Build history of the part. All positions in model axes, mm. Round coordinates to 2 decimals unless told otherwise and drop trailing zeros. Write each loop counter-clockwise with the first axis right and the second up, starting at its lowest first coordinate (ties: lowest second). Pieces come first, ordered by that corner, then holes.
1) Flat gauge pins, fed straight in: pin 1 (1.5 mm diameter, centred on x = 62.5, y = 0.5, fed in from +Z); pin 2 (2.5 mm diameter, centred on x = -95, z = 0, fed in from -Y). Where does each tip first touch, or does it go through?
2) Saw through at B-B (x = -119). Write the cut outline in (y, z), plus the area to 3 significant figures.
3) Saw through at C-C (z = 106). Write the cut outline in (x, y).
4) Wall check: probe 1 along X at (y, z) = (1.25, 0.5); probe 2 along Z at (x, y) = (-95, 0.75); probe 3 along X at (y, z) = (1.6, -45). Give the ranges that are in metal, low to high.
5) Saw through at A-A (y = 2.15). State how many separate pieces and enclosed holes the cut face has, plus the area to 3 significant figures.
from build123d import *

# Parameters (mm, degrees)
SKETCH1_R           = 150
SKETCH1_R_2         = 2.45
SKETCH1_R_3         = 1.45
BOSS_EXTRUDE1_DEPTH = 3


with BuildPart() as part:
    # Sketch1 → Boss-Extrude1 (new body)
    with BuildSketch(Plane(origin=(0, 0, 0), x_dir=(1, 0, 0), z_dir=(0, 1, 0))):
        with Locations(Location((0, 0, 0), (0, 0, 270))):
            Circle(SKETCH1_R)
        with Locations(Location((0, 10, 0), (0, 0, 270))):
            Circle(SKETCH1_R_2, mode=Mode.SUBTRACT)
        with Locations(Location((0, -10, 0), (0, 0, 270))):
            Circle(SKETCH1_R_2, mode=Mode.SUBTRACT)
        with Locations(Location((45, 0, 0), (0, 0, 270))):
            Circle(SKETCH1_R_3, mode=Mode.SUBTRACT)
        with Locations(Location((95, 0, 0), (0, 0, 270))):
            Circle(SKETCH1_R_3, mode=Mode.SUBTRACT)
        with Locations(Location((0, -45, 0), (0, 0, 270))):
            Circle(SKETCH1_R_3, mode=Mode.SUBTRACT)
        with Locations(Location((0, -95, 0), (0, 0, 270))):
            Circle(SKETCH1_R_3, mode=Mode.SUBTRACT)
        with Locations(Location((-95, 0, 0), (0, 0, 270))):
            Circle(SKETCH1_R_3, mode=Mode.SUBTRACT)
        with Locations(Location((-45, 0, 0), (0, 0, 270))):
            Circle(SKETCH1_R_3, mode=Mode.SUBTRACT)
        with Locations(Location((0, 95, 0), (0, 0, 270))):
            Circle(SKETCH1_R_3, mode=Mode.SUBTRACT)
        with Locations(Location((0, 45, 0), (0, 0, 270))):
            Circle(SKETCH1_R_3, mode=Mode.SUBTRACT)
    extrude(amount=BOSS_EXTRUDE1_DEPTH)


solid = part.part
Evaluation:
1. pin 1: stops at z = 136.7
1. pin 2: passes through
2. outline: (0, -91.32) - (3, -91.32) - (3, 91.32) - (0, 91.32) - close
2. area: 548 mm2
3. outline: (-106.13, 0) - (106.13, 0) - (106.13, 3) - (-106.13, 3) - close
4. probe 1: x = -150 to -96.36, -93.64 to -46.36, -43.64 to 43.64, 46.36 to 93.64, 96.36 to 150
4. probe 2: z = -116.08 to -1.45, 1.45 to 116.08
4. probe 3: x = -143.09 to -1.45, 1.45 to 143.09
5. separate pieces: 1
5. enclosed holes: 10
5. area: 70,600 mm2
